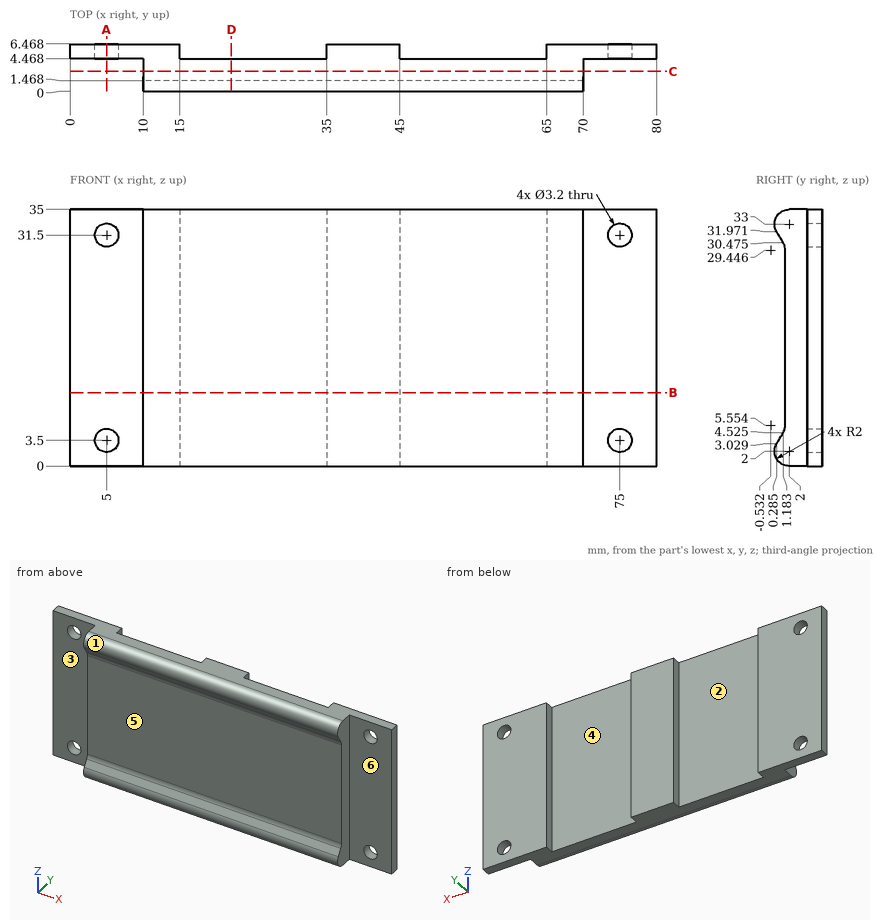
Design review of the part shown in the three views and the two pictorial views. Dimensions are in mm from the part's minimum x, y and z. A direction names the side the tool comes from. Coordinates: 2 decimals unless noted, no trailing zeros. Write each loop counter-clockwise with the first axis right and the second up, starting at its lowest first coordinate (ties: lowest second). Pieces come first, ordered by that corner, then holes. Notation, with made-up numbers: (73.5, 63.5) - (132.5, 63.5) arc R8 cw to (132.5, 68.5) - close; hole circle Ø3 at (47, 52.5). An arc over 180 degrees is marked (long way). Write item = value, one per line.
(1) For line 1 (Z direction, x = 5, y = 5.5); line 2 (X direction, y = 6, z = 8); line 3 (X direction, y = 5.5, z = 3.5), list the stretches that pass through material, from the lowest coordinate up. Write a range as [from, to].
Result sheet:
line_1 = [0, 1.9], [5.1, 29.9], [33.1, 35]
line_2 = [0, 15], [35, 45], [65, 80]
line_3 = [0, 3.4], [6.6, 15], [35, 45], [65, 73.4], [76.6, 80]
(2) Consider section C-C, the plane y = 2.75. Give the boundary of the cut face in (x, z), then the cut area to 3 significant figures.
Result sheet:
outline = (10, 0) - (70, 0) - (70, 35) - (10, 35) - close
area = 2,100 mm^2
(3) Mouldability with a two-part tool opening along X and no side actions: class the marked faces 1 and 2 as pulls with the +X half, pulls with the -X half, needs draft (parallel to the pull), parting line crosses it, or undercut.
Result sheet:
face_1 = needs draft
face_2 = undercut
(4) Consider section D-D, the plane x = 22. Give the boundary of the cut face in (y, z) (1 decimal), then the cut area to 3 significant figures.
Result sheet:
outline = (0.3, 3) arc R2 ccw to (2, 0) - (4.5, 0) - (4.5, 35) - (2, 35) arc R2 ccw to (0.3, 32) - (1.2, 30.5) arc R2 cw to (1.5, 29.4) - (1.5, 5.6) arc R2 cw to (1.2, 4.5) - close
area = 114 mm^2
(5) Consider section B-B, the plane z = 10. Give the boundary of the cut face in (x, y), then the cut area to 3 significant figures.
Result sheet:
outline = (0, 4.47) - (10, 4.47) - (10, 1.47) - (70, 1.47) - (70, 4.47) - (80, 4.47) - (80, 6.47) - (65, 6.47) - (65, 4.47) - (45, 4.47) - (45, 6.47) - (35, 6.47) - (35, 4.47) - (15, 4.47) - (15, 6.47) - (0, 6.47) - close
area = 260 mm^2
(6) For P1, Ø3, axis at x = 7, z = 20, coming from the -Y side; P2, Ø3, axis at x = 21, y = 1.5, coming from the -Z side; P3, Ø1, axis at y = 1, z = 22.5, coming from the +X side; P4, Ø2, axis at y = 2.5, z = 24, coming from the -X side, all flat-tipped, find the tip position at first contact; note any pin that passes through.
Result sheet:
P1 = 4.47
P2 = 0
P3 = 70
P4 = 10
(7) Consider section A-A, the plane x = 5. Give the boundary of the cut face in (y, z).
Result sheet:
outline = (4.47, 0) - (6.47, 0) - (6.47, 1.9) - (4.47, 1.9) - close; (4.47, 5.1) - (6.47, 5.1) - (6.47, 29.9) - (4.47, 29.9) - close; (4.47, 33.1) - (6.47, 33.1) - (6.47, 35) - (4.47, 35) - close
(8) Machinability: for the marked faces 3, 4, 5 and 6, which of the approach directions +Z, -Z, +X, -X, +Y, -Y give a long, thin tool a straight path to every point of the face, cutting with its end or side? Answer none if there is none.
Result sheet:
face_3 = +Z, -Z, -X, -Y
face_4 = +Z, -Z, +Y
face_5 = +X, -X, -Y
face_6 = +Z, -Z, +X, -Y
